Input: part model. Units: mm. Frame: model coordinates. Face numbers are marked on the shaded views. A direction names the side the tool comes from. Give positions to 0.01 mm unless a question says otherwise; leave off trailing zeros. Write each loop counter-clockwise with the first axis right and the second up, starting at its lowest first coordinate (ties: lowest second). Pieces come first, ordered by that corner, then holes. Notation, with made-up numbers: (-9.75, 89) -> (44.25, 89) arc R10 ccw to (44.25, 108) -> close; hole circle Ø6 at (70.5, 43.25). An arc over 180 degrees is marked (long way). Return JSON: item names as keys, results as strings. Group by question number.
Item 1: Section B-B, the plane x = -7. Return loops of the section in (y, z).
Item 2: Pin query (flat end, axial travel): P1, Ø0.9, axis at x = 1, z = 1, coming from the +Y side; P2, Ø1.5, axis at y = 0, z = 1.5, coming from the -X side; P3, Ø1.5, axis at x = -7.5, z = 2, coming from the -Y side. Return the tip coordinate at first contact, or that it passes through.
Item 3: Mould query, pull axis Y, two halves, no side actions, for the marked faces 4, 5 and 6. Classes: released by +Y, released by -Y, zero draft, split by the parting line, or undercut.
Item 4: Line query: line 1 (Y direction, x = 10.5, z = 2.75); line 2 (X direction, y = 2.5, z = 1.3); line 3 (X direction, y = 5.75, z = 2.25). Output: solid intervals per line, ascending. Write a range as [from, to].
Item 5: Section C-C, the plane y = -0.75. Return loops of the section in (x, z), then the cut area to 3 significant figures.
Item 6: Section A-A, the plane z = 2.5. Return loops of the section in (x, y).
Item 7: Set-up query: the marked faces 1, 2 and 3. Return all of +Z, -Z, +X, -X, +Y, -Y with unobstructed straight access to the full face (end or side cutting, diameter ignored); none if empty.
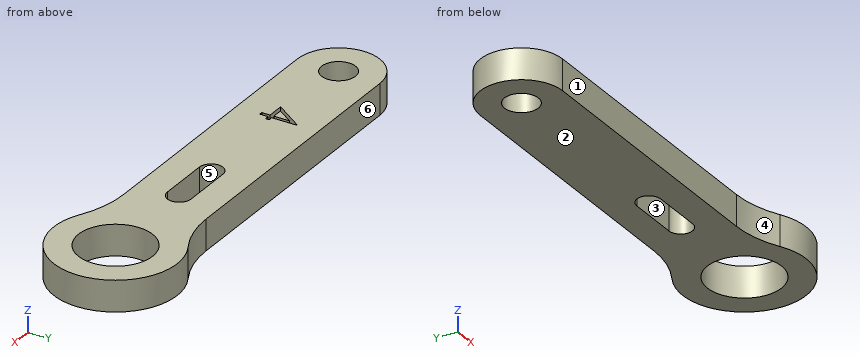
from build123d import *

# Parameters (mm, degrees)
SKETCH_1_R          = 1.65
SKETCH_1_R_2        = 3.6
EXTRUDE_1_DEPTH     = 3
CUT_EXTRUDE_1_DEPTH = 1


with BuildPart() as part:
    # 草图1 → 凸台-拉伸1 (new body)
    with BuildSketch(Plane.XY.offset(3)):
        with BuildLine():
            Line((15.64082314, 8), (-11.611020882, 8))
            ThreePointArc((-11.611020882, 8), (-15.611020882, 4), (-11.611020882, 0))
            Line((-11.611020882, 0), (15.646226321, 0))
            ThreePointArc((15.646226321, 0), (18.142339112, -0.316538794), (20.480428598, -1.246115814))
            ThreePointArc((20.480428598, -1.246115814), (29.372947843, 4.002649377), (20.478403544, 9.247982185))
            ThreePointArc((20.478403544, 9.247982185), (18.13880451, 8.317020651), (15.64082314, 8))
        make_face()
        with Locations(Location((-11.619385977, 4.000182729, 0), (0, 0, 180))):
            Circle(SKETCH_1_R, mode=Mode.SUBTRACT)
        with Locations(Location((23.379334845, 4.0005, 0), (0, 0, 180))):
            Circle(SKETCH_1_R_2, mode=Mode.SUBTRACT)
        with BuildLine():
            Line((13.380380647, 2.850266624), (8.378847398, 2.850266624))
            ThreePointArc((8.378847398, 2.850266624), (7.228847398, 4.000266624), (8.378847398, 5.150266624))
            Line((8.378847398, 5.150266624), (13.380380647, 5.150266624))
            ThreePointArc((13.380380647, 5.150266624), (14.530380647, 4.000266624), (13.380380647, 2.850266624))
        make_face(mode=Mode.SUBTRACT)
    extrude(amount=-EXTRUDE_1_DEPTH)

    # 草图2 → 切除-拉伸1 (cut)
    with BuildSketch(Plane.XY.offset(3)):
        Polygon((-2.014219225, 5.919649072), (-1.950417142, 5.919649072), (-1.950417142, 3.496572149), (-1.546570988, 3.496572149), (-1.546570988, 3.13759779), (-1.950417142, 3.13759779), (-1.950417142, 2.329905482), (-2.264519706, 2.329905482), (-2.264519706, 3.13759779), (-3.924776116, 3.13759779), align=None)
        Polygon((-2.264519706, 3.496572149), (-2.264519706, 5.0166042), (-3.307788937, 3.496572149), align=None, mode=Mode.SUBTRACT)
    extrude(amount=-CUT_EXTRUDE_1_DEPTH, mode=Mode.SUBTRACT)


solid = part.part
Answer below:
{
 "1": {"outline": "(0, 0) -> (8, 0) -> (8, 3) -> (0, 3) -> close"},
 "2": {"P1": "stops at y = 8", "P2": "stops at x = -13.94", "P3": "stops at y = 0"},
 "3": {"face 4": "released by -Y", "face 5": "undercut", "face 6": "released by +Y"},
 "4": {"line 1": "y = [0, 2.85], [5.15, 8]", "line 2": "x = [-15.32, -12.31], [-10.93, 20.11], [26.65, 29.18]", "line 3": "x = [-15.21, -2.13], [-1.95, 20.23], [26.53, 29.11]"},
 "5": {"outline": "(19.45, 0) -> (27.03, 0) -> (27.03, 3) -> (19.45, 3) -> close", "area": "22.8 mm2"},
 "6": {"outline": "(-11.61, 0) -> (15.65, 0) arc R10 cw to (20.48, -1.25) arc R5.99 ccw (long way) to (20.48, 9.25) arc R10 cw to (15.64, 8) -> (-11.61, 8) arc R4 ccw to start; (-3.31, 3.5) -> (-2.26, 3.5) -> (-2.26, 5.02) -> close; hole circle Ø3.3 at (-11.62, 4); hole (-3.92, 3.14) -> (-2.26, 3.14) -> (-2.26, 2.33) -> (-1.95, 2.33) -> (-1.95, 3.14) -> (-1.55, 3.14) -> (-1.55, 3.5) -> (-1.95, 3.5) -> (-1.95, 5.92) -> (-2.01, 5.92) -> close; hole (8.38, 2.85) -> (13.38, 2.85) arc R1.15 ccw to (13.38, 5.15) -> (8.38, 5.15) arc R1.15 ccw to start; hole circle Ø7.2 at (23.38, 4)"},
 "7": {"face 1": "+Z, -Z, -X, -Y", "face 2": "-Z, +X, -X, +Y, -Y", "face 3": "+Z, -Z"}
}
